```python
from build123d import *

# Parameters (mm, degrees)
SKETCH1_W           = 3.3
SKETCH1_H           = 9.5
BOSS_EXTRUDE1_DEPTH = 7
FILLET1_R           = 1.5
SKETCH2_W           = 2
SKETCH2_H           = 6
CUT_EXTRUDE1_DEPTH  = 7


with BuildPart() as part:
    # Sketch1 → Boss-Extrude1 (new body)
    with BuildSketch(Plane.XY):
        Rectangle(SKETCH1_W, SKETCH1_H)
    extrude(amount=BOSS_EXTRUDE1_DEPTH)

    # Fillet1
    fillet1_edges = [part.edges().sort_by_distance(p)[0] for p in [
        (1.65, -4.75, 3.5),
        (-1.65, -4.75, 3.5),
        (-1.65, 4.75, 3.5),
        (1.65, 4.75, 3.5),
    ]]
    fillet(fillet1_edges, radius=FILLET1_R)

    # Sketch2 → Cut-Extrude1 (cut)
    with BuildSketch(Plane.XY.offset(7)):
        Rectangle(SKETCH2_W, SKETCH2_H)
    extrude(amount=-CUT_EXTRUDE1_DEPTH, mode=Mode.SUBTRACT)


solid = part.part
```
For this review, take the finished solid that the model builds, in its own axes (mm). A direction names the side the tool comes from. Coordinates: 2 decimals unless noted, no trailing zeros. Order: outer loops, then holes, each group sorted by start corner. A loop starts at its lowest first (then second) coordinate and runs counter-clockwise, first axis right, second up. Notation, with made-up numbers: (63.5, -14.5) -> (73.5, -14.5) arc R21 cw to (73.5, 15.5) -> close; hole circle Ø2 at (-3, 50). An arc over 180 degrees is marked (long way). Use CSV: the item, a comma, the result in double quotes. Start each with the question number.
Item 1: For faces 1 (the face through (-1, 0, 4)), 2 (the face through (-1.49, 0.07, 0)), list the 3-axis set-ups (+Z, -Z, +X, -X, +Y, -Y) from which the entire face can be reached by the end or side of a thin tool; tool diameter is ignored.
Item 2: Insertion check: pin 1 (1 mm diameter, centred on x = 0, y = 3.5, fed in from -Z). The pin has a flat end and moves straight along its axis. Give the tip position at first contact, or say it passes through.
Item 3: We need section B-B, the plane z = 2.75. Give the boundary of the cut face in (x, y), then the cut area to 3 significant figures.
Item 4: Wall thickness on probe 1 along X at (y, z) = (-1.75, 2.75); probe 2 along Y at (x, z) = (0.2, 0.5): over which ranges is each line inside the solid? List them lowest first.
Item 5: We need section C-C, the plane x = 0.5. Give the boundary of the cut face in (y, z).
Item 6: We need section D-D, the plane x = -1.4. Give the boundary of the cut face in (y, z).
Item 7: Draft analysis for pull direction X (two halves, no side actions). For faces 3 (the face through (1.22, 4.3, 3.55)), 4 (the face through (-1.49, 0.07, 7)), 5 (the face through (0, -3, 4)), state which applies: pulls with the +X half, pulls with the -X half, needs draft (parallel to the pull), parting line crosses it, or undercut.
Item 8: We need section A-A, the plane y = 1.5. Give the boundary of the cut face in (x, z), then the cut area to 3 significant figures.
Derived:
1,face 1,"+Z, -Z"
1,face 2,"-Z, +X, -X, +Y, -Y"
2,pin 1,"stops at z = 0"
3,outline,"(-1.65, -3.25) arc R1.5 ccw to (-0.15, -4.75) -> (0.15, -4.75) arc R1.5 ccw to (1.65, -3.25) -> (1.65, 3.25) arc R1.5 ccw to (0.15, 4.75) -> (-0.15, 4.75) arc R1.5 ccw to (-1.65, 3.25) -> close; hole (-1, -3) -> (1, -3) -> (1, 3) -> (-1, 3) -> close"
3,area,"17.4 mm^2"
4,probe 1,"x = -1.65 to -1, 1 to 1.65"
4,probe 2,"y = -4.75 to -3, 3 to 4.75"
5,outline,"(-4.71, 0) -> (-3, 0) -> (-3, 7) -> (-4.71, 7) -> close; (3, 0) -> (4.71, 0) -> (4.71, 7) -> (3, 7) -> close"
6,outline,"(-4.08, 0) -> (4.08, 0) -> (4.08, 7) -> (-4.08, 7) -> close"
7,face 3,"pulls with the +X half"
7,face 4,"needs draft"
7,face 5,"undercut"
8,outline,"(-1.65, 0) -> (-1, 0) -> (-1, 7) -> (-1.65, 7) -> close; (1, 0) -> (1.65, 0) -> (1.65, 7) -> (1, 7) -> close"
8,area,"9.10 mm^2"
